The listing builds one solid part. Answer for the finished solid, in the listing's coordinates (mm). A direction names the side the tool comes from. Coordinates: 2 decimals unless noted, no trailing zeros. Write each loop counter-clockwise with the first axis right and the second up, starting at its lowest first coordinate (ties: lowest second). Pieces come first, ordered by that corner, then holes.
from build123d import *

# Parameters (mm, degrees)
F0_W      = 342.9
F0_H      = 330.2
F1_DEPTH  = 12.7
F2_W      = 292.1
F2_H      = 285.75
F3_DEPTH  = 12.7
F4_W      = 330.2
F4_H      = 12.7
F4_W_2    = 6.35
F4_H_2    = 260.35
F5_DEPTH  = 12.7
F6_W      = 292.1
F6_H      = 9.525
F7_DEPTH  = 12.7
F8_W      = 292.1
F8_H      = 9.525
F9_DEPTH  = 12.7
F10_W     = 9.525
F10_H     = 260.35
F11_DEPTH = 12.7
F12_W     = 9.525
F12_H     = 260.35
F13_DEPTH = 12.7


with BuildPart() as f1:
    # F0 (on Front) → F1 (new body)
    with BuildSketch(Plane.XZ):
        with Locations((171.45, 165.1)):
            Rectangle(F0_W, F0_H)
    extrude(amount=F1_DEPTH)

    # F2 (on face) → F3 (cut)
    with BuildSketch(Plane.XZ.offset(12.7)):
        with Locations((171.45, 155.575)):
            Rectangle(F2_W, F2_H)
    extrude(amount=-F3_DEPTH, mode=Mode.SUBTRACT)

    # F4 (on face) → F5 (cut)
    with BuildSketch(Plane.XZ.offset(12.7)):
        with Locations((171.45, 317.5)):
            Rectangle(F4_W, F4_H)
        with Locations((9.525, 155.575)):
            Rectangle(F4_W_2, F4_H_2)
        with Locations((333.375, 155.575)):
            Rectangle(F4_W_2, F4_H_2)
    extrude(amount=-F5_DEPTH, mode=Mode.SUBTRACT)

    # F6 (on face) → F7 (join)
    with BuildSketch(Plane.XY.offset(12.7)):
        with Locations((171.45, -7.9375)):
            Rectangle(F6_W, F6_H)
    extrude(amount=F7_DEPTH)

    # F8 (on face) → F9 (join)
    with BuildSketch(Plane(origin=(0, 0, 298.45), x_dir=(1, 0, 0), z_dir=(0, 0, -1))):
        with Locations((171.45, 7.9375)):
            Rectangle(F8_W, F8_H)
    extrude(amount=F9_DEPTH)

    # F10 (on face) → F11 (join)
    with BuildSketch(Plane(origin=(317.5, 0, 0), x_dir=(0, -1, 0), z_dir=(-1, 0, 0))):
        with Locations((7.9375, 155.575)):
            Rectangle(F10_W, F10_H)
    extrude(amount=F11_DEPTH)

    # F12 (on face) → F13 (join)
    with BuildSketch(Plane.YZ.offset(25.4)):
        with Locations((-7.9375, 155.575)):
            Rectangle(F12_W, F12_H)
    extrude(amount=F13_DEPTH)


solid = f1.part
Q1. The part is cut by section C-C, the plane x = 112.5. Write down the section's boundary in (y, z) (3 decimals), then the cut area to 3 significant figures.
Answers below:
outline: (-12.7, 0) - (0, 0) - (0, 12.7) - (-3.175, 12.7) - (-3.175, 25.4) - (-12.7, 25.4) - close; (-12.7, 285.75) - (-3.175, 285.75) - (-3.175, 298.45) - (0, 298.45) - (0, 311.15) - (-12.7, 311.15) - close; (-12.7, 323.85) - (0, 323.85) - (0, 330.2) - (-12.7, 330.2) - close
area: 645 mm2
Q2. Which of the six approach directions +Z, -Z, +X, -X, +Y, -Y give full straight-line access (tool end or side, diameter ignored) to faces 1 (the face through (169, -12.7, 16)), 2 (the face through (171, -3.175, 17)), 3 (the face through (12.7, -6, 154))?
Answers below:
face 1: +Z, -Z, +X, -X, -Y
face 2: +Y
face 3: +Y, -Y
Q3. Determine the mould class of faces 4 (the face through (342.9, -6, 163)), 5 (the face through (169, -6, 311.15)), 6 (the face through (145, 0, 300)), 7 (the face through (6.35, -6, 154)) for opening direction X: released by +X, released by -X, zero draft, split by the parting line, or undercut.
Answers below:
face 4: released by +X
face 5: undercut
face 6: zero draft
face 7: undercut
Q4. The part is cut by section A-A, the plane z = 264.5. Write down the section's boundary in (x, y) (3 decimals), then the cut area to 3 significant figures.
Answers below:
outline: (0, -12.7) - (6.35, -12.7) - (6.35, 0) - (0, 0) - close; (12.7, -12.7) - (38.1, -12.7) - (38.1, -3.175) - (25.4, -3.175) - (25.4, 0) - (12.7, 0) - close; (304.8, -12.7) - (330.2, -12.7) - (330.2, 0) - (317.5, 0) - (317.5, -3.175) - (304.8, -3.175) - close; (336.55, -12.7) - (342.9, -12.7) - (342.9, 0) - (336.55, 0) - close
area: 726 mm2
Q5. The part is cut by section B-B, the plane y = -7.5. Write down the section's boundary in (x, z), then the cut area to 3 significant figures.
Answers below:
outline: (0, 0) - (342.9, 0) - (342.9, 330.2) - (0, 330.2) - close; hole (6.35, 25.4) - (12.7, 25.4) - (12.7, 285.75) - (6.35, 285.75) - close; hole (6.35, 311.15) - (336.55, 311.15) - (336.55, 323.85) - (6.35, 323.85) - close; hole (38.1, 25.4) - (304.8, 25.4) - (304.8, 285.75) - (38.1, 285.75) - close; hole (330.2, 25.4) - (336.55, 25.4) - (336.55, 285.75) - (330.2, 285.75) - close
area: 36,300 mm2
Q6. Find the intervals of material crossed by probe 1 along Z at (x, y) = (181, -9); probe 2 along X at (y, z) = (-3, 52.5); probe 3 along X at (y, z) = (-11.25, 268.5), in increasing order.
Answers below:
probe 1: z = 0 to 25.4, 285.75 to 311.15, 323.85 to 330.2
probe 2: x = 0 to 6.35, 12.7 to 25.4, 317.5 to 330.2, 336.55 to 342.9
probe 3: x = 0 to 6.35, 12.7 to 38.1, 304.8 to 330.2, 336.55 to 342.9
